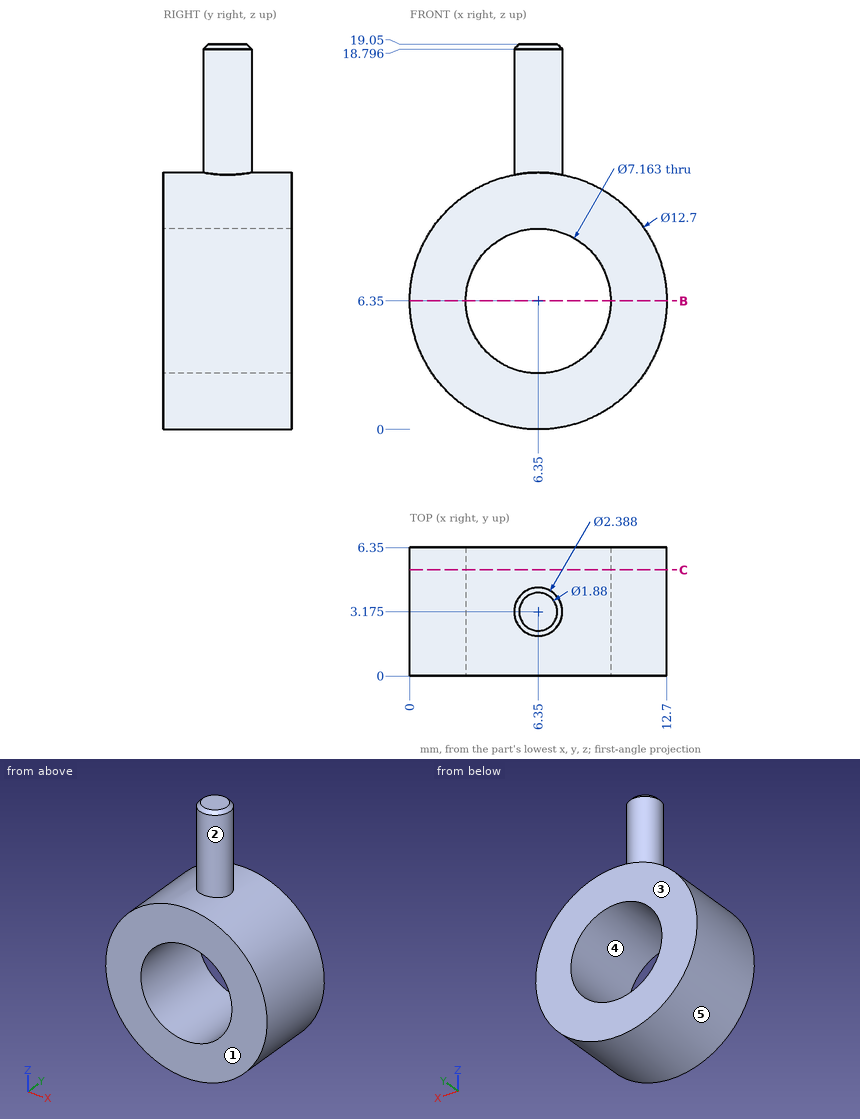
Source: three-view drawing plus pictorial views. Frame: mm from the lowest corner of the part. A direction names the side the tool comes from. Round coordinates to 2 decimals unless told otherwise and drop trailing zeros. Loops run counter-clockwise (first coordinate to the right, second up) from the corner with the lowest first, then second, coordinate; pieces in that order, holes last.
1. Access query for the marked faces 1 and 2. Directions: +Z, -Z, +X, -X, +Y, -Y. A direction counts if a zero-diameter tool reaches every point of the face in a straight line with its end or side. Return the directions, or none.
2. Contact query for flat-ended pins moving along their axis: pin 1 (5 mm diameter, centred on x = 9.5, z = 5, fed in from -Y); pin 2 (2 mm diameter, centred on y = 3.5, z = 9.5, fed in from +X) (1 decimal); pin 3 (3 mm diameter, centred on x = 11, y = 3, fed in from +Z). Output: stop coordinate, or through.
3. Ray query, L1, parallel to X at y = 4.75, z = 6.35; L2, parallel to Z at x = 4.5, y = 0.5 (1 decimal); L3, parallel to X at y = 2.5, z = 7.25 (1 decimal). Return the intervals inside material, ascending.
4. Mould query, pull axis X, two halves, no side actions, for the marked faces 3, 4 and 5. Classes: released by +X, released by -X, zero draft, split by the parting line, or undercut.
5. Section query C-C on y = 5.25. Output: boundary loops of the cut face in (x, z).
6. Section query B-B on z = 6.35. Output: boundary loops of the cut face in (x, y).
Answers below:
1. face 1: +Z, -Z, +X, -X, -Y
1. face 2: +Z
2. pin 1: stops at y = 0
2. pin 2: stops at x = 12.3
2. pin 3: stops at z = 11.86
3. L1: x = 0 to 2.77, 9.93 to 12.7
3. L2: z = 0.3 to 3.3, 9.4 to 12.4
3. L3: x = 0.1 to 2.9, 9.8 to 12.6
4. face 3: zero draft
4. face 4: undercut
4. face 5: split by the parting line
5. outline: circle Ø12.7 at (6.35, 6.35); hole circle Ø7.16 at (6.35, 6.35)
6. outline: (0, 0) - (2.77, 0) - (2.77, 6.35) - (0, 6.35) - close; (9.93, 0) - (12.7, 0) - (12.7, 6.35) - (9.93, 6.35) - close
